Read the model definition and answer for the solid it produces. Units are mm, in the model's axes. A direction names the side the tool comes from. Coordinates: 2 decimals unless noted, no trailing zeros. Loops run counter-clockwise (first coordinate to the right, second up) from the corner with the lowest first, then second, coordinate; pieces in that order, holes last. Notation, with made-up numbers: (-27, 89) -> (-23, 89) arc R9 cw to (-23, 103) -> close; hole circle Ø11 at (70.25, 55.5). An arc over 180 degrees is marked (long way). Answer as a JSON object with one key per item and string values. Group by question number.
1) Flat-ended cylindrical pins translate along their axes: P1, Ø1.5, axis at x = -16.5, y = 1.5, coming from the +Z side; P2, Ø10, axis at x = 21.5, y = -6, coming from the -Z side; P3, Ø1.3, axis at x = 29, z = 1.5, coming from the +Y side; P4, Ø1, axis at x = 30, z = 1.5, coming from the -Y side. Find the tip coordinate at first contact, or state that the pin passes through.
2) Consider probe 1 along X at (y, z) = (13.65, 2.25); probe 2 along Y at (x, z) = (-14, 2.7); probe 3 along Z at (x, y) = (29.75, 14.1). Determine where each line is inside the solid, lowest interval first. Write a range as [from, to].
3) Determine the mould class of faces 1 (the face through (14, 14, 4)), 2 (the face through (30.5, 15, 1.7)), 3 (the face through (30, -13, 4.5)) for opening direction Y: released by +Y, released by -Y, zero draft, split by the parting line, or undercut.
4) Which of the six approach directions +Z, -Z, +X, -X, +Y, -Y give full straight-line access (tool end or side, diameter ignored) to faces 4 (the face through (-5.5, 17, 3)), 5 (the face through (30.2, -15, 1.7)), 6 (the face through (-30.5, 15, 1.7))?
5) Section A-A, the plane y = -5.5 is taken. Give the vertices of the cut face in (x, z).
from build123d import *

# Parameters (mm, degrees)
SKETCH1_W           = 55
SKETCH1_H           = 40
BOSS_EXTRUDE1_DEPTH = 4.5
SKETCH2_W           = 46
SKETCH2_H           = 1.4
SKETCH2_W_2         = 55
SKETCH2_H_2         = 30
CUT_EXTRUDE1_DEPTH  = 2
CUT_EXTRUDE2_REACH  = 45.96
SKETCH3_R           = 8.5
SKETCH3_W           = 11
SKETCH3_H           = 5
SKETCH4_W           = 4.5
SKETCH4_H           = 4
BOSS_EXTRUDE2_DEPTH = 4.5
SKETCH5_R           = 0.5
CUT_EXTRUDE3_DEPTH  = 45.780017865
FILLET1_R           = 1.5
FILLET2_R           = 5
FILLET3_R           = 1
FILLET4_R           = 1


with BuildPart() as part:
    # Sketch1 → Boss-Extrude1 (new body)
    with BuildSketch(Plane.XY):
        Rectangle(SKETCH1_W, SKETCH1_H)
    extrude(amount=BOSS_EXTRUDE1_DEPTH)

    # Sketch2 → Cut-Extrude1 (cut)
    with BuildSketch(Plane.XY.offset(4.5)):
        with Locations((0, 13.3)):
            Rectangle(SKETCH2_W, SKETCH2_H)
        with Locations((0, -3.5)):
            Rectangle(SKETCH2_W_2, SKETCH2_H_2)
    extrude(amount=-CUT_EXTRUDE1_DEPTH, mode=Mode.SUBTRACT)

    # Sketch3 → Cut-Extrude2 (cut, up to next)
    with BuildSketch(Plane.XZ.offset(-14), mode=Mode.PRIVATE) as cut_extrude2_sk1:
        with Locations((-12.5, 12.75)):
            Circle(SKETCH3_R)
    cut_extrude2_tool1 = extrude(cut_extrude2_sk1.sketch, amount=-CUT_EXTRUDE2_REACH, mode=Mode.PRIVATE) & part.part
    # Sketch3 → Cut-Extrude2 (cut, up to next)
    with BuildSketch(Plane.XZ.offset(-14), mode=Mode.PRIVATE) as cut_extrude2_sk2:
        with Locations((12.5, 12.75)):
            Circle(SKETCH3_R)
    cut_extrude2_tool2 = extrude(cut_extrude2_sk2.sketch, amount=-CUT_EXTRUDE2_REACH, mode=Mode.PRIVATE) & part.part
    # Sketch3 → Cut-Extrude2 (cut, up to next)
    with BuildSketch(Plane.XZ.offset(-14), mode=Mode.PRIVATE) as cut_extrude2_sk3:
        with Locations((0, 5)):
            Rectangle(SKETCH3_W, SKETCH3_H)
    cut_extrude2_tool3 = extrude(cut_extrude2_sk3.sketch, amount=-CUT_EXTRUDE2_REACH, mode=Mode.PRIVATE) & part.part
    add(cut_extrude2_tool1.solids().sort_by_distance((-12.5, 14, 12.75))[0], mode=Mode.SUBTRACT)
    add(cut_extrude2_tool2.solids().sort_by_distance((12.5, 14, 12.75))[0], mode=Mode.SUBTRACT)
    add(cut_extrude2_tool3.solids().sort_by_distance((0, 14, 5))[0], mode=Mode.SUBTRACT)

    # Sketch4 → Boss-Extrude2 (add)
    with BuildSketch(Plane.ZY.offset(27.5)):
        with Locations((2.25, 13)):
            Rectangle(SKETCH4_W, SKETCH4_H)
        with Locations((2.25, -13)):
            Rectangle(SKETCH4_W, SKETCH4_H)
    boss_extrude2 = extrude(amount=BOSS_EXTRUDE2_DEPTH)

    # Sketch5 → Cut-Extrude3 (cut, symmetric)
    with BuildSketch(Plane.XZ.offset(-11)):
        with Locations(Location((-29.75, 2.25, 0), (0, 0, 270))):
            Circle(SKETCH5_R)
    cut_extrude3 = extrude(amount=CUT_EXTRUDE3_DEPTH, both=True, mode=Mode.SUBTRACT)

    # Mirror1: Boss-Extrude2, Cut-Extrude3 across plane
    add(boss_extrude2.mirror(Plane(origin=(0, 0, 0), x_dir=(0, 0, 1), z_dir=(1, 0, 0))))
    add(cut_extrude3.mirror(Plane(origin=(0, 0, 0), x_dir=(0, 0, 1), z_dir=(1, 0, 0))), mode=Mode.SUBTRACT)

    # Fillet1
    fillet1_edges = [part.edges().sort_by_distance(p)[0] for p in [
        (27.5, 15, 2.25),
        (27.5, -15, 1.25),
        (-27.5, 15, 2.25),
        (-27.5, -15, 1.25),
    ]]
    fillet(fillet1_edges, radius=FILLET1_R)

    # Fillet2
    # the kernel refuses this fillet: 5 mm, written as the material it takes off along each edge
    with BuildSketch(Plane(origin=(-27.5, 20, -12.061388301), x_dir=(1, 0, 0), z_dir=(0, 0, 1)), Plane(origin=(27.5, -20, -12.061388301), x_dir=(-1, 0, 0), z_dir=(0, 0, 1))) as fillet2_piece_1:
        with BuildLine():
            CenterArc((4.82455532, -5), FILLET2_R, 90, 76.657636203)
            Line((-0.040487234, -3.846153846), (-0.526991489, -3.730769231))
            ThreePointArc((-0.526991489, -3.730769231), (-0.5, -3.5), (-0.5, 0))
            Line((-0.5, 0), (0, 0.5))
            Line((0, 0.5), (4.82455532, 0.5))
            Line((4.82455532, 0.5), (4.82455532, 0))
        make_face()
    extrude(amount=28.622776602, mode=Mode.SUBTRACT)
    with BuildSketch(Plane(origin=(27.5, 20, -12.061388301), x_dir=(0.010526097592205859, -0.9999445991001099, 0), z_dir=(0, 0, 1)), Plane(origin=(-27.5, -20, -12.061388301), x_dir=(-0.010526097592205859, 0.9999445991001099, 0), z_dir=(0, 0, 1))) as fillet2_piece_2:
        with BuildLine():
            CenterArc((4.948939255, -4.876918524), FILLET2_R, 102.739251693, 76.657636203)
            Line((-0.05078374, -4.824288036), (-0.55075604, -4.819024987))
            Line((-0.55075604, -4.819024987), (-0.4999723, 0.005263049))
            Line((-0.4999723, 0.005263049), (0.005263049, 0.4999723))
            ThreePointArc((0.005263049, 0.4999723), (3.505069146, 0.463130958), (3.736109707, 0.487691852))
            Line((3.736109707, 0.487691852), (3.846366938, 0))
        make_face()
    extrude(amount=28.622776602, mode=Mode.SUBTRACT)

    # Fillet3
    fillet3_edges = [part.edges().sort_by_distance(p)[0] for p in [
        (27.5, 0, 2.5),
        (-27.5, 0, 2.5),
    ]]
    fillet(fillet3_edges, radius=FILLET3_R)

    # Fillet4
    # the kernel refuses this fillet: 1 mm, written as the material it takes off along each edge
    with BuildSketch(Plane(origin=(29, 15, 4.5), x_dir=(0, 0, -1), z_dir=(1, 0, 0))) as fillet4_piece_1:
        with BuildLine():
            CenterArc((FILLET4_R, -FILLET4_R), FILLET4_R, 90, 90)
            Line((0, -FILLET4_R), (0, 0))
            Line((0, 0), (FILLET4_R, 0))
        make_face()
    extrude(amount=5.5, mode=Mode.SUBTRACT)
    with BuildSketch(Plane(origin=(25, -15, 4.5), x_dir=(0, 0, -1), z_dir=(1, 0, 0)), Plane(origin=(-25, -15, 4.5), x_dir=(0, 1, 0), z_dir=(-1, 0, 0))) as fillet4_piece_2:
        with BuildLine():
            CenterArc((FILLET4_R, FILLET4_R), FILLET4_R, 180, 90)
            Line((0, FILLET4_R), (0, 0))
            Line((0, 0), (FILLET4_R, 0))
        make_face()
    extrude(amount=9.5, mode=Mode.SUBTRACT)
    with BuildSketch(Plane(origin=(29, 16.5, 4.5), x_dir=(0, -1, 0), z_dir=(1, 0, 0))) as fillet4_piece_3:
        with BuildLine():
            CenterArc((1.5 + FILLET4_R, FILLET4_R), FILLET4_R, 180, 90)
            Line((1.5 + FILLET4_R, 0), (1.5, 0))
            Line((1.5, 0), (1.5, FILLET4_R))
        make_face()
    revolve(axis=Axis((29, 16.5, 4.5), (0, 0, -1)), revolution_arc=76.657636203, mode=Mode.SUBTRACT)
    with BuildSketch(Plane(origin=(-29, 16.5, 4.5), x_dir=(0.9730085108210323, -0.23076923076926206, 0), z_dir=(0.23076923076926206, 0.9730085108210323, 0))) as fillet4_piece_4:
        with BuildLine():
            CenterArc((1.5 + FILLET4_R, FILLET4_R), FILLET4_R, 180, 90)
            Line((1.5 + FILLET4_R, 0), (1.5, 0))
            Line((1.5, 0), (1.5, FILLET4_R))
        make_face()
    revolve(axis=Axis((-29, 16.5, 4.5), (0, 0, -1)), revolution_arc=76.657636203, mode=Mode.SUBTRACT)
    with BuildSketch(Plane(origin=(22.67544468, 20, 4.5), x_dir=(0, 0, -1), z_dir=(-1, 0, 0)), Plane(origin=(-12.046338193, 20, 4.5), x_dir=(0, 0, -1), z_dir=(-1, 0, 0))) as fillet4_piece_5:
        with BuildLine():
            CenterArc((FILLET4_R, FILLET4_R), FILLET4_R, 180, 90)
            Line((0, FILLET4_R), (0, 0))
            Line((0, 0), (FILLET4_R, 0))
        make_face()
    extrude(amount=10.629106487, mode=Mode.SUBTRACT)
    with BuildSketch(Plane(origin=(22.67544468, 15, 4.5), x_dir=(0, 1, 0), z_dir=(-1, 0, 0))) as fillet4_piece_6:
        with BuildLine():
            CenterArc((5 - FILLET4_R, FILLET4_R), FILLET4_R, 270, 90)
            Line((5 - FILLET4_R, 0), (5, 0))
            Line((5, 0), (5, FILLET4_R))
        make_face()
    revolve(axis=Axis((22.67544468, 15, 4.5), (0, 0, -1)), revolution_arc=76.657636203, mode=Mode.SUBTRACT)
    with BuildSketch(Plane(origin=(-22.67544468, 15, 4.5), x_dir=(-0.9730085108210407, 0.2307692307692272, 0), z_dir=(-0.2307692307692272, -0.9730085108210407, 0))) as fillet4_piece_7:
        with BuildLine():
            CenterArc((5 - FILLET4_R, FILLET4_R), FILLET4_R, 270, 90)
            Line((5 - FILLET4_R, 0), (5, 0))
            Line((5, 0), (5, FILLET4_R))
        make_face()
    revolve(axis=Axis((-22.67544468, 15, 4.5), (0, 0, -1)), revolution_arc=76.657636203, mode=Mode.SUBTRACT)
    with BuildSketch(Plane(origin=(-22.67544468, -20, 4.5), x_dir=(0, 0, -1), z_dir=(1, 0, 0))) as fillet4_piece_8:
        with BuildLine():
            CenterArc((FILLET4_R, FILLET4_R), FILLET4_R, 180, 90)
            Line((0, FILLET4_R), (0, 0))
            Line((0, 0), (FILLET4_R, 0))
        make_face()
    extrude(amount=45.350889359, mode=Mode.SUBTRACT)
    with BuildSketch(Plane(origin=(-22.67544468, -15, 4.5), x_dir=(0, -1, 0), z_dir=(1, 0, 0))) as fillet4_piece_9:
        with BuildLine():
            CenterArc((5 - FILLET4_R, FILLET4_R), FILLET4_R, 270, 90)
            Line((5 - FILLET4_R, 0), (5, 0))
            Line((5, 0), (5, FILLET4_R))
        make_face()
    revolve(axis=Axis((-22.67544468, -15, 4.5), (0, 0, -1)), revolution_arc=74.223835896, mode=Mode.SUBTRACT)
    with BuildSketch(Plane(origin=(22.67544468, -15, 4.5), x_dir=(0.9623311828904709, -0.2718799265054833, 0), z_dir=(0.2718799265054833, 0.9623311828904709, 0))) as fillet4_piece_10:
        with BuildLine():
            CenterArc((5 - FILLET4_R, FILLET4_R), FILLET4_R, 270, 90)
            Line((5 - FILLET4_R, 0), (5, 0))
            Line((5, 0), (5, FILLET4_R))
        make_face()
    revolve(axis=Axis((22.67544468, -15, 4.5), (0, 0, -1)), revolution_arc=74.223835896, mode=Mode.SUBTRACT)
    with BuildSketch(Plane(origin=(12.953661807, 20, 4.5), x_dir=(0, 0, -1), z_dir=(-1, 0, 0)), Plane(origin=(-3, 20, 4.5), x_dir=(0, 0, -1), z_dir=(-1, 0, 0))) as fillet4_piece_11:
        with BuildLine():
            CenterArc((FILLET4_R, FILLET4_R), FILLET4_R, 180, 90)
            Line((0, FILLET4_R), (0, 0))
            Line((0, 0), (FILLET4_R, 0))
        make_face()
    extrude(amount=9.953661807, mode=Mode.SUBTRACT)
    with BuildSketch(Plane(origin=(-29, 15, 4.5), x_dir=(0, 0, -1), z_dir=(-1, 0, 0))) as fillet4_piece_12:
        with BuildLine():
            CenterArc((FILLET4_R, FILLET4_R), FILLET4_R, 180, 90)
            Line((0, FILLET4_R), (0, 0))
            Line((0, 0), (FILLET4_R, 0))
        make_face()
    extrude(amount=5.5, mode=Mode.SUBTRACT)


solid = part.part
Determined:
{
 "1": {"P1": "z = 2.5", "P2": "z = 0", "P3": "y = 15.15", "P4": "y = -15"},
 "2": {"probe 1": "[-32, -30.25], [-29.25, 29.25], [30.25, 32]", "probe 2": "[-20, -18.5], [11.5, 12.6], [14, 20]", "probe 3": "[0, 1.75], [2.75, 4.49]"},
 "3": {"face 1": "undercut", "face 2": "released by +Y", "face 3": "zero draft"},
 "4": {"face 4": "+Z, +Y", "face 5": "+Z, +X, -Y", "face 6": "+Z, -Z, -X, +Y"},
 "5": {"outline": "(-27.5, 0) -> (27.5, 0) -> (27.5, 1.5) arc R1 ccw to (26.5, 2.5) -> (-26.5, 2.5) arc R1 ccw to (-27.5, 1.5) -> close"}
}
